Check sheet for the drawn part. Datum: minimum x, y, z corner. Units: mm. Round coordinates to 2 decimals unless told otherwise and drop trailing zeros. Write each loop counter-clockwise with the first axis right and the second up, starting at its lowest first coordinate (ties: lowest second). Pieces come first, ordered by that corner, then holes. Notation, with made-up numbers: (57.5, 35.25) - (87.5, 35.25) arc R23 cw to (87.5, 72.25) - close; hole circle Ø6 at (22, 38). An arc over 180 degrees is marked (long way). Answer as a JSON object with one key per item and string values. Group by question number.
1) Thickness scan on line 1 (Z direction, x = 3.5, y = 32.5); line 2 (Y direction, x = 11.75, z = 11); line 3 (Z direction, x = 9, y = 44). Record the ranges inside material, lowest first.
2) Section check D-D (x = 14.5). Enter the section's corners in (y, z).
3) Section check A-A (y = 4.5). Enter the section's corners in (x, z), then the cut area to 4 significant figures.
4) Mould release check, pull along Z, two halves, no side actions. Record for the marked faces 1, 2 and 3: +Z half, -Z half, draft (parallel to the pull), parting line (faces both ways), or undercut.
5) Go/stop test with flat-tipped pins: pin 1 Ø2 at (x, y) = (9, 41) entering from -Z; pin 2 Ø8 at (x, z) = (4.5, 57.5) entering from -Y; pin 3 Ø1.5 at (x, y) = (11.5, 48.5) entering from -Z. Record where each tip stops, or that it passes through.
6) Section check C-C (y = 32.5). Enter the section's corners in (x, z).
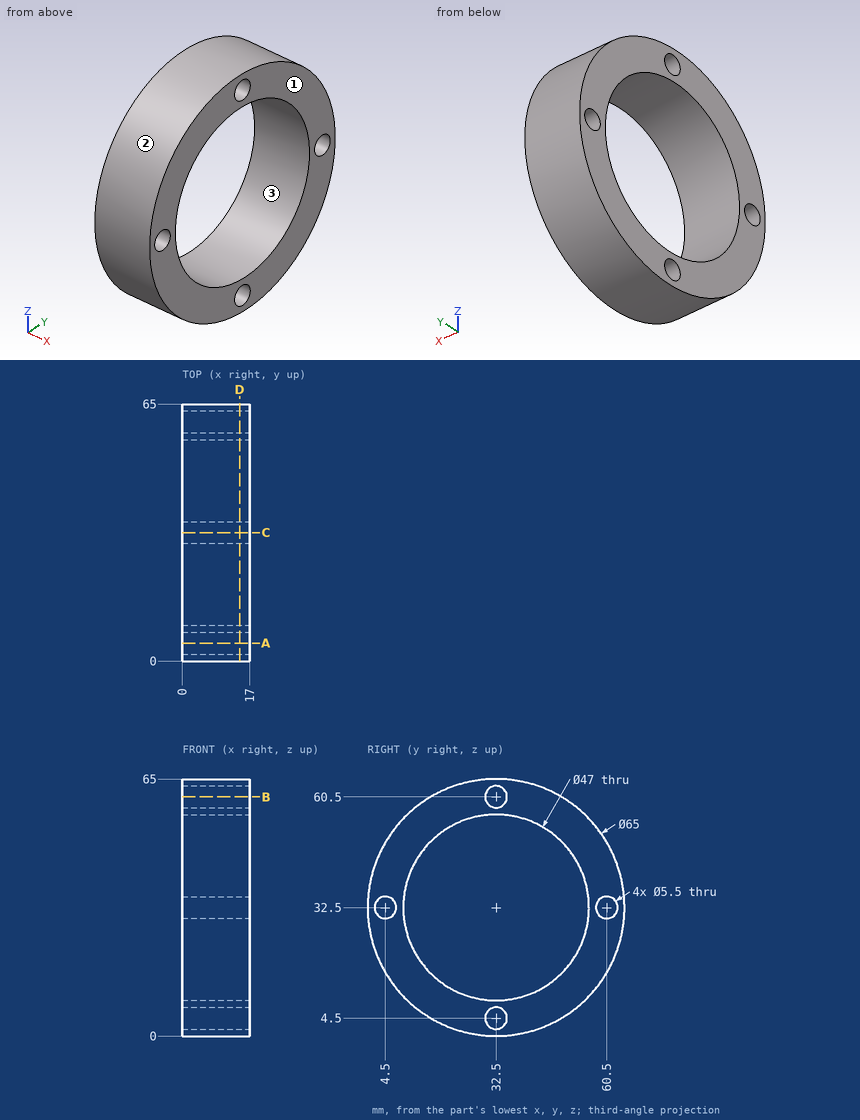
Returned:
{
 "1": {"line 1": "0 to 1.75, 7.25 to 9, 56 to 57.75, 63.25 to 65", "line 2": "8.13 to 23.01, 41.99 to 56.87", "line 3": "2.1 to 12.01, 52.99 to 62.9"},
 "2": {"outline": "circle Ø65 at (32.5, 32.5); hole circle Ø5.5 at (4.5, 32.5); hole circle Ø47 at (32.5, 32.5); hole circle Ø5.5 at (32.5, 4.5); hole circle Ø5.5 at (32.5, 60.5); hole circle Ø5.5 at (60.5, 32.5)"},
 "3": {"outline": "(0, 16) - (17, 16) - (17, 29.75) - (0, 29.75) - close; (0, 35.25) - (17, 35.25) - (17, 49) - (0, 49) - close", "area": "467.5 mm2"},
 "4": {"face 1": "draft", "face 2": "parting line", "face 3": "undercut"},
 "5": {"pin 1": "z = 0.88", "pin 2": "y = 7.7", "pin 3": "z = 3.8"},
 "6": {"outline": "(0, 0) - (17, 0) - (17, 1.75) - (0, 1.75) - close; (0, 7.25) - (17, 7.25) - (17, 9) - (0, 9) - close; (0, 56) - (17, 56) - (17, 57.75) - (0, 57.75) - close; (0, 63.25) - (17, 63.25) - (17, 65) - (0, 65) - close"}
}
